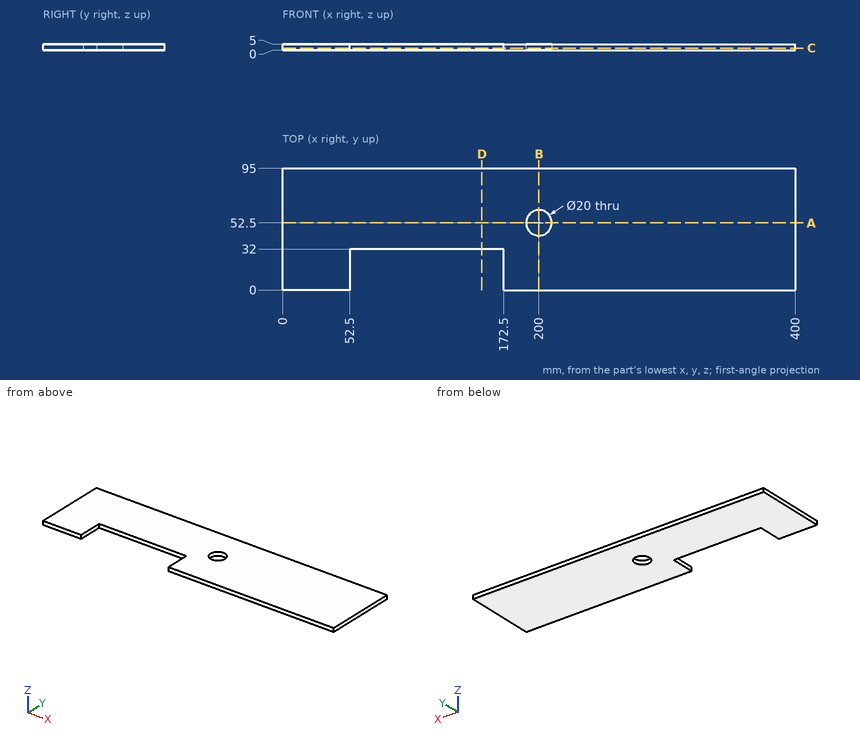
Study the drawing (mm; zero at the part's minimum x, y, z) and answer. Give positions to 0.01 mm unless a question says otherwise; leave off trailing zeros. Write each loop counter-clockwise with the first axis right and the second up, starting at its lowest first coordinate (ties: lowest second). Pieces come first, ordered by that corner, then holes. Notation, with made-up numbers: (-2.75, 1.25) - (35.25, 1.25) arc R16 cw to (35.25, 16.25) - close; hole circle Ø4 at (69, 81.25). An arc over 180 degrees is marked (long way). Use CSV: the item, a comma, the result in double quotes. Start each with the question number.
(1) Find section C-C (z = 1.7). Give the vertices of the cut face in (x, y), plus the area to 3 significant figures.
(2) Find section B-B (x = 200). Give the vertices of the cut face in (y, z).
(3) Consider line 1 along Y through (x, z) = (200, 2.5); line 2 along X through (y, z) = (24, 0.95); line 3 along Y through (x, z) = (102.5, 4.4). Determine where each line is inside the solid, lowest interval first.
(4) Find section A-A (y = 52.5). Give the vertices of the cut face in (x, z), plus the area to 3 significant figures.
(5) Find section D-D (x = 155.5). Give the vertices of the cut face in (y, z).
(6) Given P1, Ø2.5, axis at x = 126.5, z = 2, coming from the -Y side, flat-ended and moving along its own axis, determine where the tip first touches the part or whether it passes through.
Findings below:
1,outline,"(0, 0) - (52.5, 0) - (52.5, 32) - (172.5, 32) - (172.5, 0) - (400, 0) - (400, 95) - (0, 95) - close; hole circle Ø20 at (200, 52.5)"
1,area,"33,800 mm2"
2,outline,"(0, 0) - (42.5, 0) - (42.5, 5) - (0, 5) - close; (62.5, 0) - (95, 0) - (95, 5) - (62.5, 5) - close"
3,line 1,"0 to 42.5, 62.5 to 95"
3,line 2,"0 to 52.5, 172.5 to 400"
3,line 3,"32 to 95"
4,outline,"(0, 0) - (190, 0) - (190, 5) - (0, 5) - close; (210, 0) - (400, 0) - (400, 5) - (210, 5) - close"
4,area,"1,900 mm2"
5,outline,"(32, 0) - (95, 0) - (95, 5) - (32, 5) - close"
6,P1,"y = 32"
